from build123d import *

# Parameters (mm, degrees)
K_TOWNIK_STALOWY_35_X_35_X_5_1_DEPTH = 300
SZKIC2_R                             = 5
WYTNIJ_WYCI_GNI_CIE1_DEPTH           = 304.521004216


with BuildPart() as part:
    # Sketch1 → Kątownik stalowy 35 X 35 X 5(1) (new body)
    with BuildSketch(Plane(origin=(0, 0, 0), x_dir=(0, 0, -1), z_dir=(1, 0, 0))):
        with BuildLine():
            Line((0, 0), (0, 35))
            ThreePointArc((0, 35), (3.535533906, 33.535533906), (5, 30))
            Line((5, 30), (5, 10))
            ThreePointArc((5, 10), (6.464466094, 6.464466094), (10, 5))
            Line((10, 5), (30, 5))
            ThreePointArc((30, 5), (33.535533906, 3.535533906), (35, 0))
            Line((35, 0), (0, 0))
        make_face()
    extrude(amount=K_TOWNIK_STALOWY_35_X_35_X_5_1_DEPTH)

    # Szkic2 → Wytnij-wyciągnięcie1 (cut, through all)
    with BuildSketch(Plane(origin=(0, 0, -5), x_dir=(-1, 0, 0), z_dir=(0, 0, -1))):
        with Locations(Location((-270, 20, 0), (0, 0, 90))):
            Circle(SZKIC2_R)
        with Locations(Location((-30, 20, 0), (0, 0, 90))):
            Circle(SZKIC2_R)
    extrude(amount=-WYTNIJ_WYCI_GNI_CIE1_DEPTH, mode=Mode.SUBTRACT)


solid = part.part
Work out the finished part from the listing and answer in its coordinate system (mm). A direction names the side the tool comes from. Coordinates: 2 decimals unless noted, no trailing zeros. Write each loop counter-clockwise with the first axis right and the second up, starting at its lowest first coordinate (ties: lowest second). Pieces come first, ordered by that corner, then holes.
1. Consider line 1 along X through (y, z) = (20, -3.7); line 2 along Z through (x, y) = (254, 9.5); line 3 along Y through (x, z) = (181, -23.5). Determine where each line is inside the solid, lowest interval first.
Results list:
line 1: x = 0 to 25, 35 to 265, 275 to 300
line 2: z = -5.03 to 0
line 3: y = 0 to 5
2. The part is cut by section A-A, the plane y = 20. Write down the section's boundary in (x, z).
Results list:
outline: (0, -5) - (25, -5) - (25, 0) - (0, 0) - close; (35, -5) - (265, -5) - (265, 0) - (35, 0) - close; (275, -5) - (300, -5) - (300, 0) - (275, 0) - close
3. The part is cut by section B-B, the plane x = 30. Write down the section's boundary in (y, z).
Results list:
outline: (0, -35) arc R5 ccw to (5, -30) - (5, -10) arc R5 cw to (10, -5) - (15, -5) - (15, 0) - (0, 0) - close; (25, -5) - (30, -5) arc R5 ccw to (35, 0) - (25, 0) - close
4. The part is cut by section D-D, the plane z = -15. Write down the section's boundary in (x, y), and give its area (3 significant figures).
Results list:
outline: (0, 0) - (300, 0) - (300, 5) - (0, 5) - close
area: 1,500 mm2
5. Flat-ended cylindrical pins translate along their axes: pin 1 (12 mm diameter, centred on x = 161, y = 8, fed in from -Z); pin 2 (4 mm diameter, centred on x = 145.5, y = 28.5, fed in from -Z); pin 3 (5 mm diameter, centred on x = 133, z = -28.5, fed in from +Y). Find the tip coordinate at first contact, or state that the pin passes through.
Results list:
pin 1: stops at z = -34.58
pin 2: stops at z = -5
pin 3: stops at y = 5
6. For a pull along Y with two mould halves and no side action, classify faces 1 (the cylindrical face through (148, 4, -33)), 2 (the cylindrical face through (274.957, 19.349, -2.535)), 3 (the flat face through (148, 0, -18)), 4 (the flat face through (148, 17, 0)) as +Y half, -Y half, draft (parallel to the pull), parting line (faces both ways), or undercut.
Results list:
face 1: +Y half
face 2: undercut
face 3: -Y half
face 4: draft
7. The part is cut by section C-C, the plane x = 74. Write down the section's boundary in (y, z), and give its area (3 significant figures).
Results list:
outline: (0, -35) arc R5 ccw to (5, -30) - (5, -10) arc R5 cw to (10, -5) - (30, -5) arc R5 ccw to (35, 0) - (0, 0) - close
area: 320 mm2
8. For faces 5 (the flat face through (300, 4.6, -9.8)), 6 (the flat face through (148, 20, -5)), determine the directions among +Z, -Z, +X, -X, +Y, -Y from which every point of the face is accessible in a straight line to the end or side of a thin tool.
Results list:
face 5: +Z, -Z, +X, +Y, -Y
face 6: -Z, +X, -X, +Y
